The listing builds one solid part. Answer for the finished solid, in the listing's coordinates (mm). A direction names the side the tool comes from. Round coordinates to 2 decimals unless told otherwise and drop trailing zeros. Write each loop counter-clockwise with the first axis right and the second up, starting at its lowest first coordinate (ties: lowest second). Pieces come first, ordered by that corner, then holes.
from build123d import *

# Parameters (mm, degrees)
SKETCH2_R                = 1.1
BOSS_EXTRUDE1_DEPTH      = 5
BOSS_EXTRUDE2_DEPTH      = 1.5
BOSS_EXTRUDE2_DEPTH_BACK = 1
SKETCH4_W                = 65
SKETCH4_H                = 20
SKETCH4_R                = 1.55
FILLET1_R                = 2
FILLET2_R                = 2
FILLET3_DEPTH            = 5
FILLET3_START            = -46.68249578
FILLET3_2_DEPTH          = 13.56249578
FILLET3_START_2          = 5
FILLET3_3_DEPTH          = 3
FILLET4_START            = -44.68249568
FILLET4_DEPTH            = 11.56249568
FILLET4_START_2          = -46.68249588
FILLET4_2_DEPTH          = 2.0000002
FILLET4_START_3          = -2
FILLET4_3_DEPTH          = 2
BOSS_EXTRUDE3_START      = -5
BOSS_EXTRUDE3_DEPTH      = 5


with BuildPart() as part:
    # Sketch2 → Boss-Extrude1 (new body)
    with BuildSketch(Plane.XY):
        with BuildLine():
            Line((20.317595566, -31.62), (26.767401765, -31.62))
            ThreePointArc((26.767401765, -31.62), (28.079366857, -31.746249368), (29.343182309, -32.120364071))
            ThreePointArc((29.343182309, -32.120364071), (29.713933476, -32.121815396), (29.983758291, -31.867545651))
            Line((29.983758291, -31.867545651), (30.409159516, -30.952682564))
            ThreePointArc((30.409159516, -30.952682564), (30.957401765, -31.242707116), (31.482691519, -31.572486555))
            Line((31.482691519, -31.572486555), (30.903097457, -32.398326366))
            ThreePointArc((30.903097457, -32.398326366), (30.817805806, -32.759136383), (31.004438274, -33.07949065))
            ThreePointArc((31.004438274, -33.07949065), (33.576739296, -37.51647451), (32.365115584, -42.5))
            ThreePointArc((32.365115584, -42.5), (27.155948468, -45.369019687), (21.656472124, -43.105735361))
            Line((21.656472124, -43.105735361), (20.317595566, -41.62))
            Line((20.317595566, -41.62), (20.317595566, -31.62))
        make_face()
        with Locations(Location((26.767401765, -38.5, 0), (0, 0, 180))):
            Circle(SKETCH2_R, mode=Mode.SUBTRACT)
    extrude(amount=BOSS_EXTRUDE1_DEPTH)

    # Sketch4 → Boss-Extrude2 (add, two sides: drawn at the far end of the back side and taken through both)
    with BuildSketch(Plane.ZY.offset(-20.317595566).offset(-BOSS_EXTRUDE2_DEPTH_BACK)):
        with Locations((-1.5, -43.12)):
            Rectangle(SKETCH4_W, SKETCH4_H)
        with Locations((21, -43.12)):
            Circle(SKETCH4_R, mode=Mode.SUBTRACT)
        with Locations((-24, -43.12)):
            Circle(SKETCH4_R, mode=Mode.SUBTRACT)
    extrude(amount=BOSS_EXTRUDE2_DEPTH + BOSS_EXTRUDE2_DEPTH_BACK)

    # Fillet1
    # the kernel refuses this fillet: 2 mm, written as the material it adds along each edge
    with BuildSketch(Plane(origin=(20.317595566, -33.12, 5), x_dir=(0, 1, 0), z_dir=(0, 0, -1))) as fillet1_piece_1:
        with BuildLine():
            CenterArc((1.948957881, -1.948957881), FILLET1_R, 102.972239886, 64.055520228)
            Line((0, -1.5), (0, 0))
            Line((0, 0), (1.5, 0))
        make_face()
    extrude(amount=5)

    # Fillet2
    fillet2_edges = [part.edges().sort_by_distance(p)[0] for p in [
        (20.317595566, -31.62, 2.5),
    ]]
    fillet(fillet2_edges, radius=FILLET2_R)

    # Fillet3: read off the stored shape, not the designer's step
    # Fillet3 outline → Fillet3 (add)
    with BuildSketch(Plane.XY):
        with BuildLine():
            Line((21.317595566, -42.729688082), (21.317595566, -46.68249578))
            ThreePointArc((21.317595566, -46.68249578), (22.211694747, -45.01606745), (24.094578944, -44.839591325))
            ThreePointArc((24.094578944, -44.839591325), (22.780138954, -44.106793672), (21.656472124, -43.105735361))
            Line((21.656472124, -43.105735361), (21.317595566, -42.729688082))
        make_face()
    extrude(amount=FILLET3_DEPTH)

    # Fillet3 2 outline → Fillet3 2 (add)
    with BuildSketch(Plane(origin=(0, 0, 0), x_dir=(1, 0, 0), z_dir=(0, 1, 0)).offset(FILLET3_START)):
        with BuildLine():
            Line((21.317595566, -5), (21.317595566, -7))
            ThreePointArc((21.317595566, -7), (21.903382004, -5.585786438), (23.317595566, -5))
            Line((23.317595566, -5), (21.317595566, -5))
        make_face()
    extrude(amount=FILLET3_2_DEPTH)

    # Fillet3 3 outline → Fillet3 3 (cut)
    with BuildSketch(Plane.XY.offset(FILLET3_START_2)):
        with BuildLine():
            ThreePointArc((24.094578944, -44.839591325), (22.211694747, -45.01606745), (21.317595566, -46.68249578))
            Line((21.317595566, -46.68249578), (25, -46.68249578))
            Line((25, -46.68249578), (25, -45.221324143))
            Line((25, -45.221324143), (24.094578944, -44.839591325))
        make_face()
    extrude(amount=FILLET3_3_DEPTH, mode=Mode.SUBTRACT)

    # Fillet4: read off the stored shape, not the designer's step
    # Fillet4 outline → Fillet4 (add)
    with BuildSketch(Plane(origin=(0, 0, 0), x_dir=(1, 0, 0), z_dir=(0, 1, 0)).offset(FILLET4_START)):
        with BuildLine():
            ThreePointArc((22.317595566, 0), (21.610488785, 0.292893219), (21.317595566, 1))
            Line((21.317595566, 1), (21.317595566, 0))
            Line((21.317595566, 0), (22.317595566, 0))
        make_face()
    extrude(amount=FILLET4_DEPTH)

    # Fillet4 2 outline → Fillet4 2 (add)
    with BuildSketch(Plane(origin=(0, 0, 0), x_dir=(1, 0, 0), z_dir=(0, 1, 0)).offset(FILLET4_START_2)):
        with BuildLine():
            ThreePointArc((22.317595566, 0), (21.610488785, 0.292893219), (21.317595566, 1))
            Line((21.317595566, 1), (21.317595566, 0))
            Line((21.317595566, 0), (22.317595566, 0))
        make_face()
    extrude(amount=FILLET4_2_DEPTH)

    # Fillet4 3 outline → Fillet4 3 (cut)
    with BuildSketch(Plane.XY.offset(FILLET4_START_3)):
        with BuildLine():
            ThreePointArc((24, -44.802515943), (22.169729909, -45.044691019), (21.317595566, -46.68249578))
            Line((21.317595566, -46.68249578), (24, -46.68249588))
            Line((24, -46.68249588), (24, -44.802515943))
        make_face()
    extrude(amount=FILLET4_3_DEPTH, mode=Mode.SUBTRACT)

    # Sketch5 → Boss-Extrude3 (add)
    with BuildSketch(Plane(origin=(0, 0, 5), x_dir=(-1, 0, 0), z_dir=(0, 0, 1)).offset(BOSS_EXTRUDE3_START)):
        with BuildLine():
            Line((-33.69491521, 33.784710246), (-32.869075399, 34.364304307))
            ThreePointArc((-32.869075399, 34.364304307), (-32.508265382, 34.449595959), (-32.187911115, 34.262963491))
            Line((-32.187911115, 34.262963491), (-31.321885711, 34.762963491))
            Line((-31.321885711, 34.762963491), (-32.28101229, 36.424219456))
            Line((-32.28101229, 36.424219456), (-33.147037694, 35.924219456))
            ThreePointArc((-33.147037694, 35.924219456), (-33.145586368, 35.553468289), (-33.399856114, 35.283643474))
            Line((-33.399856114, 35.283643474), (-34.314719201, 34.858242249))
            ThreePointArc((-34.314719201, 34.858242249), (-34.024694648, 34.31), (-33.69491521, 33.784710246))
        make_face()
    extrude(amount=BOSS_EXTRUDE3_DEPTH)


solid = part.part
1. Section A-A on z = -24 is taken. Determine the outline of the cut face in (x, y), plus the area to 4 significant figures.
Geometry says:
outline: (18.82, -53.12) - (21.32, -53.12) - (21.32, -44.67) - (18.82, -44.67) - close; (18.82, -41.57) - (21.32, -41.57) - (21.32, -33.12) - (18.82, -33.12) - close
area: 42.25 mm2
2. Section B-B on y = -38.5 is taken. Determine the outline of the cut face in (x, z).
Geometry says:
outline: (18.82, -34) - (21.32, -34) - (21.32, -1) arc R1 cw to (22.32, 0) - (25.67, 0) - (25.67, 5) - (23.32, 5) arc R2 cw to (21.32, 7) - (21.32, 31) - (18.82, 31) - close; (27.87, 0) - (33.65, 0) - (33.65, 5) - (27.87, 5) - close
3. Section C-C on y = -43.12 is taken. Determine the outline of the cut face in (x, z).
Geometry says:
outline: (18.82, -34) - (21.32, -34) - (21.32, -25.55) - (18.82, -25.55) - close; (18.82, -22.45) - (21.32, -22.45) - (21.32, -1) arc R1 cw to (22.32, 0) - (31.87, 0) - (31.87, 5) - (23.32, 5) arc R2 cw to (21.32, 7) - (21.32, 19.45) - (18.82, 19.45) - close; (18.82, 22.55) - (21.32, 22.55) - (21.32, 31) - (18.82, 31) - close
4. Straight lines are drawn through the part: line 1 along Y through (x, z) = (20.35, -24); line 2 along X through (y, z) = (-38.5, 2.35); line 3 along Y through (x, z) = (19.75, -5.5). For each, find the intervals that lie inside material, in ascending order.
Geometry says:
line 1: y = -53.12 to -44.67, -41.57 to -33.12
line 2: x = 18.82 to 25.67, 27.87 to 33.65
line 3: y = -53.12 to -33.12
5. Section D-D on z = 26 is taken. Determine the outline of the cut face in (x, y).
Geometry says:
outline: (18.82, -53.12) - (21.32, -53.12) - (21.32, -33.12) - (18.82, -33.12) - close
6. A tool of negligible diameter and unlimited length cuts with its end or side. For faces 1 (the face through (28.061, -31.743, 2.465)), 2 (the face through (31.624, -33.627, 2.465)), 3 (the face through (24, -31.62, 2)), 4 (the face through (20, -33.12, -17)), from which of +Z, -Z, +X, -X, +Y, -Y can it reach the whole face along a straight path? Write none if from no direction.
Geometry says:
face 1: +Z, -Z, +Y
face 2: +Z, -Z
face 3: +Z, -Z, -X, +Y
face 4: -Z, +X, -X, +Y
7. For a pull along Y with two mould halves and no side action, classify faces 5 (the face through (21.318, -43, -2)), 6 (the face through (20, -33.12, 18)), 7 (the face through (20.085, -44.633, -24.336)) as released by +Y, released by -Y, zero draft, split by the parting line, or undercut.
Geometry says:
face 5: zero draft
face 6: released by +Y
face 7: undercut
8. Given pin 1 (1.1 mm diameter, centred on x = 21, z = -19, fed in from +Y); pin 2 (2 mm diameter, centred on x = 24, y = -41.5, fed in from +Z); pin 3 (8 mm diameter, centred on y = -33.5, z = 24.5, fed in from +X), each flat-ended and moving along its own axis, determine where each tip first touches the part or whether it passes through.
Geometry says:
pin 1: stops at y = -33.12
pin 2: stops at z = 5.03
pin 3: stops at x = 21.32
